from build123d import *

# Parameters (mm, degrees)
SKETCH2_W               = 92
SKETCH2_H               = 30
BOSS_EXTRUDE1_DEPTH     = 16
SKETCH3_W               = 1
SKETCH3_H               = 30
BOSS_EXTRUDE2_DEPTH     = 3
SKETCH6_OUTSIDE_W       = 40.724
SKETCH6_OUTSIDE_H       = 51.724
CUT_EXTRUDE1_DEPTH      = 95.578010129
SKETCH7_R               = 1.6
CUT_EXTRUDE2_DEPTH      = 51.960769225
CUT_EXTRUDE3_DEPTH      = 51.0999002
CUT_EXTRUDE3_DEPTH_BACK = 1
SKETCH8_R               = 3.1
SHELL3_OUTLINE_W        = 88
SHELL3_OUTLINE_H        = 14
SHELL3_DEPTH            = 14
SHELL3_2_OUTLINE_W      = 88
SHELL3_2_OUTLINE_H      = 3
SHELL3_2_DEPTH          = 10.937428747
SHELL3_3_DEPTH          = 1
SHELL3_START            = -44
SHELL3_4_DEPTH          = 88
SHELL3_START_2          = 1
SHELL3_5_DEPTH          = 2.266756081
SKETCH9_R               = 1.35
SKETCH9_W               = 15.7
SKETCH9_H               = 8.2
CUT_EXTRUDE4_DEPTH      = 52.980765673
SKETCH10_R              = 1.15
SKETCH10_W              = 15.7
SKETCH10_H              = 7.4
CUT_EXTRUDE5_DEPTH      = 52.980765673
SKETCH11_R              = 1.55
CUT_EXTRUDE6_DEPTH      = 10
FILLET1_R               = 2
FILLET3_R               = 5


with BuildPart() as part:
    # Sketch2 → Boss-Extrude1 (new body)
    with BuildSketch(Plane.XY):
        Rectangle(SKETCH2_W, SKETCH2_H)
    extrude(amount=BOSS_EXTRUDE1_DEPTH)

    # Sketch3 → Boss-Extrude2 (add)
    with BuildSketch(Plane.XY):
        with Locations((45.5, 0)):
            Rectangle(SKETCH3_W, SKETCH3_H)
    boss_extrude2 = extrude(amount=-BOSS_EXTRUDE2_DEPTH)

    # Mirror1: Boss-Extrude2 across plane
    add(boss_extrude2.mirror(Plane(origin=(0, 0, 0), x_dir=(0, 0, 1), z_dir=(1, 0, 0))))

    # Sketch6 outside → Cut-Extrude1 (cut, through all)
    with BuildSketch(Plane(origin=(46, 0, 0), x_dir=(0, 0, -1), z_dir=(1, 0, 0))):
        with Locations((-6.5, 0)):
            Rectangle(SKETCH6_OUTSIDE_W, SKETCH6_OUTSIDE_H)
        Polygon((-12.5, 6), (-16, 6), (-16, -12), (-13.247984009, -12), (-12.5, -15), (3, -15), (3, 15), (-3, 15), (-3, 8), align=None, mode=Mode.SUBTRACT)
    extrude(amount=-CUT_EXTRUDE1_DEPTH, mode=Mode.SUBTRACT)

    # Sketch7 → Cut-Extrude2 (cut, through all)
    with BuildSketch(Plane.XY):
        with Locations((-15, 11)):
            Circle(SKETCH7_R)
        with Locations((15, 11)):
            Circle(SKETCH7_R)
    extrude(amount=CUT_EXTRUDE2_DEPTH, mode=Mode.SUBTRACT)

    # Sketch8 → Cut-Extrude3 (cut, two sides: drawn at the far end of the back side and taken through both)
    with BuildSketch(Plane.XY.offset(3).offset(-CUT_EXTRUDE3_DEPTH_BACK)):
        with Locations(Location((15, 11, 0), (0, 0, 255.407449398))):
            Circle(SKETCH8_R)
        with Locations(Location((-15, 11, 0), (0, 0, 255.407449398))):
            Circle(SKETCH8_R)
    extrude(amount=CUT_EXTRUDE3_DEPTH + CUT_EXTRUDE3_DEPTH_BACK, mode=Mode.SUBTRACT)

    # Shell3: read off the stored shape, not the designer's step
    # Shell3 outline → Shell3 (cut)
    with BuildSketch(Plane.XY):
        with Locations((0, -3)):
            Rectangle(SHELL3_OUTLINE_W, SHELL3_OUTLINE_H)
    extrude(amount=SHELL3_DEPTH, mode=Mode.SUBTRACT)

    # Shell3 2 outline → Shell3 2 (cut)
    with BuildSketch(Plane.XY):
        with Locations((0, -11.5)):
            Rectangle(SHELL3_2_OUTLINE_W, SHELL3_2_OUTLINE_H)
    extrude(amount=SHELL3_2_DEPTH, mode=Mode.SUBTRACT)

    # Shell3 3 outline → Shell3 3 (cut)
    with BuildSketch(Plane.XY):
        with BuildLine():
            Line((-19.691481642, 13), (-44, 13))
            Line((-44, 13), (-44, 4))
            Line((-44, 4), (44, 4))
            Line((44, 4), (44, 13))
            Line((44, 13), (19.691481642, 13))
            ThreePointArc((19.691481642, 13), (15, 5.9), (10.308518358, 13))
            Line((10.308518358, 13), (-10.308518358, 13))
            ThreePointArc((-10.308518358, 13), (-15, 5.9), (-19.691481642, 13))
        make_face()
    extrude(amount=SHELL3_3_DEPTH, mode=Mode.SUBTRACT)

    # Shell3 4 outline → Shell3 4 (cut)
    with BuildSketch(Plane.YZ.offset(SHELL3_START)):
        Polygon((4, 1), (6.377211806, 1), (4, 12.291756081), align=None)
        Polygon((-10, 10.937428747), (-10, 11.685412756), (-13, 10.937428747), align=None)
    extrude(amount=SHELL3_4_DEPTH, mode=Mode.SUBTRACT)

    # Shell3 5 outline → Shell3 5 (add)
    with BuildSketch(Plane.XY.offset(SHELL3_START_2)):
        with BuildLine():
            Line((17.154026303, 6.377211806), (12.845973697, 6.377211806))
            ThreePointArc((12.845973697, 6.377211806), (15, 5.9), (17.154026303, 6.377211806))
        make_face()
        with BuildLine():
            ThreePointArc((-17.154026303, 6.377211806), (-15, 5.9), (-12.845973697, 6.377211806))
            Line((-12.845973697, 6.377211806), (-17.154026303, 6.377211806))
        make_face()
    extrude(amount=SHELL3_5_DEPTH)

    # Sketch9 → Cut-Extrude4 (cut, through all)
    with BuildSketch(Plane.XY.offset(16)):
        with Locations((9.55, -3)):
            Circle(SKETCH9_R)
        with Locations((30.45, -3)):
            Circle(SKETCH9_R)
        with Locations((20, -3)):
            Rectangle(SKETCH9_W, SKETCH9_H)
    extrude(amount=-CUT_EXTRUDE4_DEPTH, mode=Mode.SUBTRACT)

    # Sketch10 → Cut-Extrude5 (cut, through all)
    with BuildSketch(Plane.XY.offset(16)):
        with Locations((-29.55, -3)):
            Circle(SKETCH10_R)
        with Locations((-10.45, -3)):
            Circle(SKETCH10_R)
        with Locations((-20, -3)):
            Rectangle(SKETCH10_W, SKETCH10_H)
    extrude(amount=-CUT_EXTRUDE5_DEPTH, mode=Mode.SUBTRACT)

    # Sketch11 → Cut-Extrude6 (cut)
    with BuildSketch(Plane.XZ.offset(15)):
        with Locations(Location((-20, 5, 0), (0, 0, 270))):
            Circle(SKETCH11_R)
        with Locations(Location((20, 5, 0), (0, 0, 270))):
            Circle(SKETCH11_R)
    extrude(amount=-CUT_EXTRUDE6_DEPTH, mode=Mode.SUBTRACT)

    # Fillet1
    fillet1_edges = [part.edges().sort_by_distance(p)[0] for p in [
        (0, -12, 16),
        (0, 6, 16),
    ]]
    fillet(fillet1_edges, radius=FILLET1_R)

    # Fillet3
    # the kernel refuses this fillet: 5 mm, written as the material it adds along each edge
    with BuildSketch(Plane(origin=(24.361401242, 8, 3), x_dir=(0, -0.20601048104984168, 0.978549784986749), z_dir=(-1, 0, 0))) as fillet3_piece_1_section:
        with BuildLine():
            CenterArc((FILLET3_R * 0.811394096787, FILLET3_R), FILLET3_R, 191.88865804, 78.11134196)
            Line((-FILLET3_R * 0.1671556882, FILLET3_R * 0.79398951895), (0, 0))
            Line((0, 0), (FILLET3_R * 0.811394096787, 0))
        make_face()
    fillet3_piece_1 = extrude(amount=48.722802484, mode=Mode.PRIVATE)
    fillet3_piece_1 = fillet3_piece_1 - Plane(origin=(-15, 11, 3), x_dir=(-0.2519435379319081, -0.967741935484018, 0), z_dir=(0, 0, -1)) * Cylinder(3.1, 114, mode=Mode.PRIVATE)
    fillet3_piece_1 = fillet3_piece_1 - Plane(origin=(15, 11, 3), x_dir=(-0.2519435379319081, -0.967741935484018, 0), z_dir=(0, 0, -1)) * Cylinder(3.1, 114, mode=Mode.PRIVATE)
    add(fillet3_piece_1)
    with BuildSketch(Plane(origin=(46, 8, 3), x_dir=(0, -0.20601048104984168, 0.978549784986749), z_dir=(-1, 0, 0))) as fillet3_piece_2_section:
        with BuildLine():
            CenterArc((FILLET3_R * 0.811394096787, FILLET3_R), FILLET3_R, 191.88865804, 78.11134196)
            Line((-FILLET3_R * 0.1671556882, FILLET3_R * 0.79398951895), (0, 0))
            Line((0, 0), (FILLET3_R * 0.811394096787, 0))
        make_face()
    fillet3_piece_2 = extrude(amount=40.361401242, mode=Mode.PRIVATE)
    fillet3_piece_2 = fillet3_piece_2 - Plane(origin=(15, 11, 3), x_dir=(-0.2519435379319081, -0.967741935484018, 0), z_dir=(0, 0, -1)) * Cylinder(3.1, 97, mode=Mode.PRIVATE)
    add(fillet3_piece_2)
    with BuildSketch(Plane(origin=(-5.638598758, 8, 3), x_dir=(0, -0.20601048104984168, 0.978549784986749), z_dir=(-1, 0, 0))) as fillet3_piece_3_section:
        with BuildLine():
            CenterArc((FILLET3_R * 0.811394096787, FILLET3_R), FILLET3_R, 191.88865804, 78.11134196)
            Line((-FILLET3_R * 0.1671556882, FILLET3_R * 0.79398951895), (0, 0))
            Line((0, 0), (FILLET3_R * 0.811394096787, 0))
        make_face()
    fillet3_piece_3 = extrude(amount=40.361401242, mode=Mode.PRIVATE)
    fillet3_piece_3 = fillet3_piece_3 - Plane(origin=(-15, 11, 3), x_dir=(-0.2519435379319081, -0.967741935484018, 0), z_dir=(0, 0, -1)) * Cylinder(3.1, 97, mode=Mode.PRIVATE)
    add(fillet3_piece_3)


solid = part.part
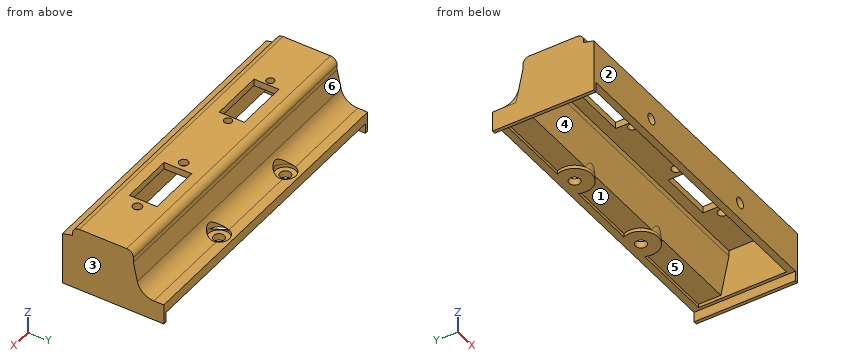
The model under review builds one solid part; all positions refer to its coordinate system, in mm. Face numbers are marked on the shaded views. A direction names the side the tool comes from. Round coordinates to 2 decimals unless told otherwise and drop trailing zeros. Order: outer loops, then holes, each group sorted by start corner. A loop starts at its lowest first (then second) coordinate and runs counter-clockwise, first axis right, second up. Notation, with made-up numbers: (22, 49) -> (38, 49) arc R12 ccw to (38, 68) -> close; hole circle Ø11 at (23.5, 36.5). An arc over 180 degrees is marked (long way). Write item = value, one per line. Start each with the question number.
Item 1: Consider section A-A on x = -29.55. Write out the cut boundary in (y, z).
Item 2: Consider section D-D on z = 9.5. Write out the cut boundary in (x, y).
Item 3: Clearance check with flat-ended pins moving along their axes: pin 1 Ø5 at (x, y) = (-15, 11) entering from -Z; pin 2 Ø3 at (x, y) = (9.55, -3) entering from +Z; pin 3 Ø3 at (x, y) = (28, 6.5) entering from +Z; pin 4 Ø2 at (x, y) = (8.5, 7) entering from -Z. State where each tip first meets the part, or that it passes through.
Item 4: For the marked faces 5 and 6, list the 3-axis set-ups (+Z, -Z, +X, -X, +Y, -Y) from which the entire face can be reached by the end or side of a thin tool; tool diameter is ignored.
Item 5: Consider section C-C on y = -3. Count the separate pieces of the cut face and the enclosed holes in it, plus the area to 3 significant figures.
Item 6: Consider section B-B on x = -7. Write out the cut boundary in (y, z).
Item 7: Mouldability with a two-part tool opening along X and no side actions: class the marked faces 1, 2, 3 and 4 as released by +X, released by -X, zero draft, split by the parting line, or undercut.
Item 8: For line 1 along X through (y, z) = (-13.35, 5); line 2 along X through (y, z) = (11, 0.8); line 3 along X through (y, z) = (-9.5, 2.25), list the stretches that pass through material, from the lowest coordinate up.
Conclusion:
q1.outline = (-15, 0) -> (-13, 0) -> (-13, 10.94) -> (-10, 11.69) -> (-10, 14) -> (-4.15, 14) -> (-4.15, 16) -> (-10, 16) arc R2 ccw to (-12, 14) -> (-12, 13.25) -> (-15, 12.5) -> close; (-1.85, 14) -> (4, 14) -> (4, 12.29) -> (6.38, 1) -> (13, 1) -> (13, 0) -> (15, 0) -> (15, 3) -> (12.06, 3) arc R5 cw to (7.16, 6.97) -> (6, 12.5) -> (6, 14) arc R2 ccw to (4, 16) -> (-1.85, 16) -> close
q2.outline = (-46, -15) -> (46, -15) -> (46, 6.63) -> (-46, 6.63) -> close; hole (-44, -13) -> (44, -13) -> (44, 4.59) -> (-44, 4.59) -> close
q3.pin_1 = 0
q3.pin_2 = 16
q3.pin_3 = 15.73
q3.pin_4 = 1
q4.face_5 = -Z
q4.face_6 = +Z, +X, -X, +Y
q5.separate_pieces = 7
q5.enclosed_holes = 0
q5.area = 163 mm2
q6.outline = (-15, 0) -> (-13, 0) -> (-13, 10.94) -> (-10, 11.69) -> (-10, 14) -> (4, 14) -> (4, 12.29) -> (6.38, 1) -> (13, 1) -> (13, 0) -> (15, 0) -> (15, 3) -> (12.06, 3) arc R5 cw to (7.16, 6.97) -> (6, 12.5) -> (6, 14) arc R2 ccw to (4, 16) -> (-10, 16) arc R2 ccw to (-12, 14) -> (-12, 13.25) -> (-15, 12.5) -> close
q7.face_1 = undercut
q7.face_2 = zero draft
q7.face_3 = released by +X
q7.face_4 = undercut
q8.line_1 = -46 to -21.55, -18.45 to 18.45, 21.55 to 46
q8.line_2 = -46 to -44, -20.1 to -16.6, -13.4 to -9.9, 9.9 to 13.4, 16.6 to 20.1, 44 to 46
q8.line_3 = -46 to -44, 44 to 46
